Here's how the part is built. I have some questions about the finished solid (model axes, mm). A direction names the side the tool comes from. Round coordinates to 2 decimals unless told otherwise and drop trailing zeros. Write each question's results on one line, items separated by ' | '. Start each with the question number.
```python
from build123d import *

# Parameters (mm, degrees)
SKETCH4_R           = 8
BOSS_EXTRUDE3_DEPTH = 1
SKETCH5_R           = 7
SKETCH5_R_2         = 6
BOSS_EXTRUDE4_DEPTH = 4.75
CUT_EXTRUDE3_START  = -3
SKETCH9_R           = 6
CUT_EXTRUDE3_DEPTH  = 3
CUT_EXTRUDE7_DEPTH  = 10
SKETCH13_R          = 2.4
CUT_EXTRUDE8_DEPTH  = 10
CUT_EXTRUDE9_START  = -6
CUT_EXTRUDE9_DEPTH  = 6
CUT_EXTRUDE10_DEPTH = 10


with BuildPart() as part:
    # Sketch4 → Boss-Extrude3 (new body)
    with BuildSketch(Plane(origin=(0, 0, 0), x_dir=(1, 0, 0), z_dir=(0, 1, 0))):
        with Locations(Location((0, 0, 0), (0, 0, 270))):
            Circle(SKETCH4_R)
    extrude(amount=BOSS_EXTRUDE3_DEPTH)

    # Sketch5 → Boss-Extrude4 (add)
    with BuildSketch(Plane(origin=(0, 1, 0), x_dir=(1, 0, 0), z_dir=(0, 1, 0))):
        with Locations(Location((0, 0, 0), (0, 0, 270))):
            Circle(SKETCH5_R)
        with Locations(Location((0, 0, 0), (0, 0, 270))):
            Circle(SKETCH5_R_2, mode=Mode.SUBTRACT)
    extrude(amount=BOSS_EXTRUDE4_DEPTH)

    # Sketch6 → Revolve4 (revolve)
    with BuildSketch(Plane.XY, mode=Mode.PRIVATE) as revolve4_sk:
        Polygon((0, 5.75), (7, 5.75), (6, 7), (0, 7), align=None)
    revolve(revolve4_sk.sketch.rotate(Axis((0, 5.75, 0), (0, 1, 0)), 90), axis=Axis((0, 5.75, 0), (0, 1, 0)))

    # Sketch9 → Cut-Extrude3 (cut)
    with BuildSketch(Plane(origin=(0, 7, 0), x_dir=(1, 0, 0), z_dir=(0, 1, 0)).offset(CUT_EXTRUDE3_START)):
        with Locations(Location((0, 0, 0), (0, 0, 270))):
            Circle(SKETCH9_R)
    extrude(amount=CUT_EXTRUDE3_DEPTH, mode=Mode.SUBTRACT)

    # Sketch11 → Cut-Extrude7 (cut)
    with BuildSketch(Plane.XY):
        Polygon((0, 2.175), (2.007816798, 3.373213723), (0, 4.575), (-2.009525275, 3.375), align=None)
    extrude(amount=CUT_EXTRUDE7_DEPTH, mode=Mode.SUBTRACT)

    # Sketch13 → Cut-Extrude8 (cut)
    with BuildSketch(Plane(origin=(0, 1, 0), x_dir=(1, 0, 0), z_dir=(0, 1, 0))):
        with Locations(Location((0, 0, 0), (0, 0, 270))):
            Circle(SKETCH13_R)
    extrude(amount=-CUT_EXTRUDE8_DEPTH, mode=Mode.SUBTRACT)

    # Sketch14 → Revolve5 (revolve)
    with BuildSketch(Plane.XY):
        Polygon((6, 7), (6, 5.75), (7, 5.75), (8.08473241, 7), align=None)
    revolve(axis=Axis((0, 5.75, 0), (0, 1, 0)))

    # Sketch15 → Cut-Extrude9 (cut)
    with BuildSketch(Plane(origin=(0, 7, 0), x_dir=(1, 0, 0), z_dir=(0, 1, 0)).offset(CUT_EXTRUDE9_START)):
        with BuildLine():
            Line((-5.191534566, -6.197650119), (-4.871861689, -3.502137017))
            ThreePointArc((-4.871861689, -3.502137017), (-6, 0), (-4.871861689, 3.502137017))
            Line((-4.871861689, 3.502137017), (-6.564616348, 4.718973441))
            ThreePointArc((-6.564616348, 4.718973441), (-8.02152969, -1.008939827), (-5.191534566, -6.197650119))
        make_face()
    extrude(amount=CUT_EXTRUDE9_DEPTH, mode=Mode.SUBTRACT)

    # Sketch16 → Cut-Extrude10 (cut)
    with BuildSketch(Plane(origin=(0, 0, 0), x_dir=(0, 0, -1), z_dir=(1, 0, 0))):
        with BuildLine():
            ThreePointArc((0.6, 3.375), (0.424264069, 3.799264069), (0, 3.975))
            Line((0, 3.975), (0, 2.775))
            ThreePointArc((0, 2.775), (0.424264069, 2.950735931), (0.6, 3.375))
        make_face()
        with BuildLine():
            Line((0, 2.775), (0, 3.975))
            ThreePointArc((0, 3.975), (-0.6, 3.375), (0, 2.775))
        make_face()
    extrude(amount=CUT_EXTRUDE10_DEPTH, mode=Mode.SUBTRACT)


solid = part.part
```
(1) I want a section at A-A on x = -1. Give the number of separate pieces and of enclosed holes in the cut face, and give its area (3 significant figures).
(2) Please list where these lines run through material, in increasing order: line 1 (Z direction, x = 0, y = 5.25); line 2 (X direction, y = 0.65, z = 0); line 3 (Y direction, x = -5.25, z = 3.5).
(3) On a 3-axis mill with a long thin cutter (end or side, diameter ignored), from which of +Z, -Z, +X, -X, +Y, -Y can I reach the whole of each face in a straight line? I mean faces 1 (the cylindrical face through (-7.81, 0.49, -1.73)), 2 (the cylindrical face through (5.848, 3.342, -3.847)), 3 (the flat face through (-4.963, 3.958, 4.27)). Say none if no direction works.
(4) If we mould it in two halves opening along Y, with no side actions, what happens to faces 4 (the flat face through (6.2, 7, 0.6)), 5 (the flat face through (-5.33, 3.96, -3.83)), 6 (the conical face through (7.183, 5.967, -0.275)), 7 (the flat face through (2, 0, 2))? For each: pulls with the +Y half, pulls with the -Y half, needs draft (parallel to the pull), parting line crosses it, or undercut.
(5) I'm going to push flat-ended pins straight in: pin 1 Ø4.5 at (x, z) = (0, 0) entering from +Y; pin 2 Ø2 at (y, z) = (5.5, -4) entering from +X; pin 3 Ø4 at (x, z) = (1.5, -0.5) entering from +Y; pin 4 Ø2 at (x, y) = (-6, 2.5) entering from +Z. Where does each tip first touch, or does it pass through?
Solutions:
1) separate pieces: 3 | enclosed holes: 0 | area: 23.8 mm^2
2) line 1: -7 to -6, 6 to 7 | line 2: -8 to -2.4, 2.4 to 8 | line 3: 0 to 1
3) face 1: -Y | face 2: none | face 3: -X, +Y
4) face 4: pulls with the +Y half | face 5: needs draft | face 6: undercut | face 7: pulls with the -Y half
5) pin 1: through | pin 2: x = 6.67 | pin 3: y = 1 | pin 4: z = 4.9
